```python
from build123d import *

# Parameters (mm, degrees)
SKETCH1_W           = 119
SKETCH1_H           = 40
SKETCH1_R           = 11.5
BOSS_EXTRUDE1_DEPTH = 3
SKETCH2_W           = 26
SKETCH2_H           = 40
SKETCH2_W_2         = 8
BOSS_EXTRUDE2_DEPTH = 1.5


with BuildPart() as part:
    # Sketch1 → Boss-Extrude1 (new body)
    with BuildSketch(Plane(origin=(0, 0, 0), x_dir=(1, 0, 0), z_dir=(0, 1, 0))):
        Rectangle(SKETCH1_W, SKETCH1_H)
        with Locations((-39.5, 0)):
            Circle(SKETCH1_R, mode=Mode.SUBTRACT)
    extrude(amount=BOSS_EXTRUDE1_DEPTH)

    # Sketch2 → Boss-Extrude2 (add)
    with BuildSketch(Plane(origin=(0, 3, 0), x_dir=(1, 0, 0), z_dir=(0, 1, 0))):
        with Locations((-14.3, 0)):
            Rectangle(SKETCH2_W, SKETCH2_H)
        with Locations((-55.5, 0)):
            Rectangle(SKETCH2_W_2, SKETCH2_H)
    extrude(amount=BOSS_EXTRUDE2_DEPTH)


solid = part.part
```
The listing builds one solid part. Answer for the finished solid, in the listing's coordinates (mm). A direction names the side the tool comes from. Give positions to 0.01 mm unless a question says otherwise; leave off trailing zeros. Order: outer loops, then holes, each group sorted by start corner. A loop starts at its lowest first (then second) coordinate and runs counter-clockwise, first axis right, second up. Notation, with made-up numbers: M 79.5,67 L 96.5,67 A31 ccw 96.5,92 Z; hole C 71.25,7 d8. An arc over 180 degrees is marked long. Put each result on its own line as item: value. Start each with the question number.
Item 1: Flat-ended cylindrical pins translate along their axes: P1, Ø14, axis at x = -39.5, z = 0, coming from the -Y side; P2, Ø12, axis at x = -34, z = 4, coming from the +Y side. Find the tip coordinate at first contact, or state that the pin passes through.
Item 2: For a pull along X with two mould halves and no side action, classify faces 1 (the face through (-59.5, 2, 0)), 2 (the face through (-50.3, 3, -4.7)), 3 (the face through (59.5, 1, 0)) as +X half, -X half, draft (parallel to the pull), parting line (faces both ways), or undercut.
Item 3: The part is cut by section A-A, the plane x = -39.5. Determine the outline of the cut face in (y, z).
Item 4: Find the intervals of material crossed by line 1 along X through (y, z) = (3.85, 2); line 2 along Z through (x, y) = (-39.5, 1.8); line 3 along X through (y, z) = (2.2, 0), in increasing order.
Item 5: The part is cut by section C-C, the plane z = 6.5. Determine the outline of the cut face in (x, y).
Item 6: The part is cut by section D-D, the plane x = 34.5. Determine the outline of the cut face in (y, z), and give its area (3 significant figures).
Item 7: The part is cut by section B-B, the plane z = -9.5. Determine the outline of the cut face in (x, y).
Item 8: Which of the six approach directions +Z, -Z, +X, -X, +Y, -Y give full straight-line access (tool end or side, diameter ignored) to faces 4 (the face through (-14, 4.5, 0)), 5 (the face through (29, 3, 0))?
Answer key:
1. P1: passes through
1. P2: stops at y = 3
2. face 1: -X half
2. face 2: undercut
2. face 3: +X half
3. outline: M 0,-20 L 3,-20 L 3,-11.5 L 0,-11.5 Z; M 0,11.5 L 3,11.5 L 3,20 L 0,20 Z
4. line 1: x = -59.5 to -51.5, -27.3 to -1.3
4. line 2: z = -20 to -11.5, 11.5 to 20
4. line 3: x = -59.5 to -51, -28 to 59.5
5. outline: M -59.5,0 L -48.99,0 L -48.99,3 L -51.5,3 L -51.5,4.5 L -59.5,4.5 Z; M -30.01,0 L 59.5,0 L 59.5,3 L -1.3,3 L -1.3,4.5 L -27.3,4.5 L -27.3,3 L -30.01,3 Z
6. outline: M 0,-20 L 3,-20 L 3,20 L 0,20 Z
6. area: 120 mm²
7. outline: M -59.5,0 L -45.98,0 L -45.98,3 L -51.5,3 L -51.5,4.5 L -59.5,4.5 Z; M -33.02,0 L 59.5,0 L 59.5,3 L -1.3,3 L -1.3,4.5 L -27.3,4.5 L -27.3,3 L -33.02,3 Z
8. face 4: +Z, -Z, +X, -X, +Y
8. face 5: +Z, -Z, +X, +Y
